```python
from build123d import *

# Parameters (mm, degrees)
SKETCH1_W           = 150
SKETCH1_H           = 84
BOSS_EXTRUDE1_DEPTH = 63
SHELL1_T            = -3


with BuildPart() as part:
    # Sketch1 → Boss-Extrude1 (new body)
    with BuildSketch(Plane(origin=(0, 0, 0), x_dir=(1, 0, 0), z_dir=(0, 1, 0))):
        with Locations((-10.344827586, 2.773706897)):
            Rectangle(SKETCH1_W, SKETCH1_H)
    extrude(amount=-BOSS_EXTRUDE1_DEPTH)

    # Shell1
    shell1_openings = [part.faces().sort_by_distance(p)[0] for p in [
        (-10.344827586, 0, -2.773706897),
    ]]
    offset(amount=SHELL1_T, openings=shell1_openings, kind=Kind.INTERSECTION)


solid = part.part
```
Input: part model. Units: mm. Frame: model coordinates. A direction names the side the tool comes from. Round coordinates to 2 decimals unless told otherwise and drop trailing zeros. Order: outer loops, then holes, each group sorted by start corner. A loop starts at its lowest first (then second) coordinate and runs counter-clockwise, first axis right, second up. Notation, with made-up numbers: (57.5, 48) - (105.5, 48) arc R27 cw to (105.5, 69) - close; hole circle Ø3 at (-37, 17). An arc over 180 degrees is marked (long way). Answer in a Markdown table with one row per item.
Item 1: Section query B-B (x = 25.5). Return the cut outline in (y, z), then the cut area to 3 significant figures.
Model answer:
| item | result |
|---|---|
| outline | (-63, -44.77) - (0, -44.77) - (0, -41.77) - (-60, -41.77) - (-60, 36.23) - (0, 36.23) - (0, 39.23) - (-63, 39.23) - close |
| area | 612 mm² |
Item 2: Reachability of faces 1 (the flat face through (-11, -60, -3)), 2 (the flat face through (-11, -63, -3)) from +Z, -Z, +X, -X, +Y, -Y: full face, straight path, thin tool, end or side. Return the list, or none.
Model answer:
| item | result |
|---|---|
| face 1 | +Y |
| face 2 | +Z, -Z, +X, -X, -Y |
Item 3: Pin query (flat end, axial travel): pin 1 (2 mm diameter, centred on x = 14.5, z = -33.5, fed in from +Y). Return the tip coordinate at first contact, or that it passes through.
Model answer:
| item | result |
|---|---|
| pin 1 | stops at y = -60 |
Item 4: Mould query, pull axis X, two halves, no side actions, for faces 3 (the flat face through (64.655, -31, -2)), 4 (the flat face through (61.655, -30, -2)), 5 (the flat face through (-11, -31, -44.774)), 6 (the flat face through (-85.345, -31, -2)). Classes: released by +X, released by -X, zero draft, split by the parting line, or undercut.
Model answer:
| item | result |
|---|---|
| face 3 | released by +X |
| face 4 | undercut |
| face 5 | zero draft |
| face 6 | released by -X |
Item 5: Section query A-A (y = -42). Return the cut outline in (x, z).
Model answer:
| item | result |
|---|---|
| outline | (-85.34, -44.77) - (64.66, -44.77) - (64.66, 39.23) - (-85.34, 39.23) - close; hole (-82.34, -41.77) - (61.66, -41.77) - (61.66, 36.23) - (-82.34, 36.23) - close |
Item 6: Section query C-C (z = -32). Return the cut outline in (x, y), then the cut area to 3 significant figures.
Model answer:
| item | result |
|---|---|
| outline | (-85.34, -63) - (64.66, -63) - (64.66, 0) - (61.66, 0) - (61.66, -60) - (-82.34, -60) - (-82.34, 0) - (-85.34, 0) - close |
| area | 810 mm² |
Item 7: Line query: line 1 (X direction, y = -44, z = -10.5); line 2 (Z direction, x = -55.5, y = -47); line 3 (Y direction, x = -39, z = -30.5). Output: solid intervals per line, ascending.
Model answer:
| item | result |
|---|---|
| line 1 | x = -85.34 to -82.34, 61.66 to 64.66 |
| line 2 | z = -44.77 to -41.77, 36.23 to 39.23 |
| line 3 | y = -63 to -60 |
